Autodesk Inventor part; units mm, degrees
ref_plane "YZ Plane" through (0, 0, 0) normal (1, 0, 0) x (0, 1, 0)
ref_plane "XZ Plane" through (0, 0, 0) normal (0, 1, 0) x (-1, 0, 0)
ref_plane "XY Plane" through (0, 0, 0) normal (0, 0, 1) x (1, 0, 0)
sketch "スケッチ1" plane through (0, 0, 0) normal (0, 0, 1) x (1, 0, 0)
  circle A0 centre (0, 0) radius 6
  circle A1 centre (0, 0) radius 7
  dimension "d0" = 12
  dimension "d1" = 14
extrude "押し出し1" add sketch "スケッチ1" along normal blind 6
sketch "スケッチ2" plane through (0, 0, 0) normal (0, 0, -1) x (-1, 0, 0)
  circle A0 centre (0, 0) radius 7
  circle A1 centre (0, 0) radius 6
  circle A2 centre (0, 0) radius 10
  dimension "d4" = 20
extrude "押し出し2" add sketch "スケッチ2" along normal blind 1 contours A0 | A2
properties part number "オイレスフランジ付き12142006" material "アセタール樹脂、黒"
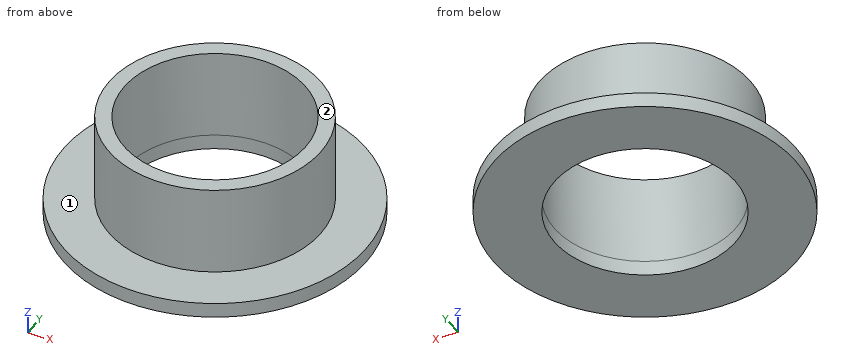
Input: part model. Units: mm. Frame: model coordinates. Face numbers are marked on the shaded views. A direction names the side the tool comes from. Coordinates: 2 decimals unless noted, no trailing zeros. Loops run counter-clockwise (first coordinate to the right, second up) from the corner with the lowest first, then second, coordinate; pieces in that order, holes last. Notation, with made-up numbers: (33.25, 22.5) -> (87.25, 22.5) arc R7 cw to (87.25, 32.5) -> close; hole circle Ø9 at (72, -4.5). An arc over 180 degrees is marked (long way). Write item = value, one per line. Start each with the question number.
Item 1: Cut plane D-D, the plane y = -6.75. Return loops of the section in (x, z), plus the area to 3 significant figures.
Item 2: First-contact query: P1, Ø1.5, axis at x = 1.5, z = 4.5, coming from the -Y side; P2, Ø12, axis at x = -7.5, y = 0, coming from the +Z side; P3, Ø3, axis at x = 3, z = 3, coming from the -Y side; P4, Ø4, axis at x = 4, z = 3.5, coming from the +Y side. Flat tips, straight axial feed; report the tip coordinate or a pass-through.
Item 3: Reachability of the marked faces 1 and 2 from +Z, -Z, +X, -X, +Y, -Y: full face, straight path, thin tool, end or side. Return the list, or none.
Item 4: Cut plane C-C, the plane z = 1.5. Return loops of the section in (x, y).
Item 5: Cut plane A-A, the plane x = 0. Return loops of the section in (y, z).
Item 6: Material intervals for line 1 (Y direction, x = 0, z = -0.25); line 2 (Z direction, x = 7, y = -3.5); line 3 (Y direction, x = 0, z = 3.55), sorted ascending.
Ans:
q1.outline = (-7.38, -1) -> (7.38, -1) -> (7.38, 0) -> (1.85, 0) -> (1.85, 6) -> (-1.85, 6) -> (-1.85, 0) -> (-7.38, 0) -> close
q1.area = 37.0 mm²
q2.P1 = -6.96
q2.P2 = 6
q2.P3 = -6.84
q2.P4 = 6.71
q3.face_1 = +Z
q3.face_2 = +Z, +X, -X, +Y, -Y
q4.outline = circle Ø14 at (0, 0); hole circle Ø12 at (0, 0)
q5.outline = (-10, -1) -> (-6, -1) -> (-6, 6) -> (-7, 6) -> (-7, 0) -> (-10, 0) -> close; (6, -1) -> (10, -1) -> (10, 0) -> (7, 0) -> (7, 6) -> (6, 6) -> close
q6.line_1 = -10 to -6, 6 to 10
q6.line_2 = -1 to 0
q6.line_3 = -7 to -6, 6 to 7
